Part model, mm, in its own coordinate system. A direction names the side the tool comes from. Coordinates: 2 decimals unless noted, no trailing zeros. Write each loop counter-clockwise with the first axis right and the second up, starting at its lowest first coordinate (ties: lowest second). Pieces come first, ordered by that corner, then holes. Notation, with made-up numbers: (-39.75, 78.25) - (18.25, 78.25) arc R18 cw to (18.25, 84.25) - close; hole circle Ø8 at (54, -38.5). An arc over 180 degrees is marked (long way). Write each question's results on one line, items separated by ' | '.
from build123d import *

# Parameters (mm, degrees)
F0_R     = 5
F1_DEPTH = 50
F3_DEPTH = 10
F4_W     = 15
F4_H     = 15
F4_R     = 5
F5_DEPTH = 10
F6_R     = 5
F7_DEPTH = 2.5
F8_SIZE  = 2.49999


# Not quite as in the source:
# - a fillet or chamfer is up to 0.001 mm smaller than in the source, because OpenCascade refuses the exact size


with BuildPart() as f1:
    # F0 (on Right) → F1 (new body)
    with BuildSketch(Plane.YZ):
        Circle(F0_R)
    extrude(amount=F1_DEPTH)

    # F2 (on face) → F3 (join)
    with BuildSketch(Plane(origin=(0, 0, 0), x_dir=(0, -1, 0), z_dir=(-1, 0, 0))):
        Polygon((11.5200223266, 0.788935313), (5.0767731403, 10.3710996435), (-6.4432491863, 9.5821643305), (-11.5200223266, -0.788935313), (-5.0767731403, -10.3710996435), (6.4432491863, -9.5821643305), align=None)
    extrude(amount=F3_DEPTH)

    # F4 (on face) → F5 (join)
    with BuildSketch(Plane.YZ.offset(50)):
        Rectangle(F4_W, F4_H)
        Circle(F4_R, mode=Mode.SUBTRACT)
    extrude(amount=-F5_DEPTH)

    # F6 (on face) → F7 (join)
    with BuildSketch(Plane.YZ.offset(50)):
        Circle(F6_R)
    extrude(amount=F7_DEPTH)

    # F8 (size 2.5 in the source; OpenCascade refuses exactly that, so slightly less here)
    f8_edges = [f1.edges().sort_by_distance(p)[0] for p in [
        (52.5, -5, 0),
    ]]
    chamfer(f8_edges, length=F8_SIZE)


solid = f1.part
(1) Flat gauge pins, fed straight in: P1, Ø4, axis at y = 1.5, z = -6.5, coming from the +X side; P2, Ø11, axis at x = 43, y = 2, coming from the +Z side; P3, Ø6, axis at y = -2.5, z = -5, coming from the +X side. Where does each tip first touch, or does it go through?
Return value:
P1: stops at x = 50.33 | P2: stops at z = 7.5 | P3: stops at x = 52.41
(2) 3-axis set-ups, long thin cutter, end or side, ignore diameter. For faces 1 (the flat face through (45, -7.5, 0)), 2 (the flat face through (40, -2, 5)), 3 (the flat face through (45, 7.5, 0)): which of +Z, -Z, +X, -X, +Y, -Y reach the whole face in a straight line?
Return value:
face 1: +Z, -Z, +X, -Y | face 2: none | face 3: +Z, -Z, +X, +Y
(3) Wall check: line 1 (X direction, y = 5.5, z = -1.5); line 2 (X direction, y = 9.5, z = -2.75); line 3 (Z direction, x = 46, y = 4.5). Give the ranges that are in metal, low to high. Write a range as from..to.
Return value:
line 1: x = -10..0, 40..50 | line 2: x = -10..0 | line 3: z = -7.5..7.5
(4) Two-plate mould, pull along X, no slides. Class faces 4 (the cylindrical face through (19.72, -1.08, -4.88)), 5 (the conical face through (52, -3, 0)), 6 (the flat face through (-4.93, 0.603, 9.982)), 7 (the flat face through (-10, 0, 0)): released by +X, released by -X, zero draft, split by the parting line, or undercut.
Return value:
face 4: undercut | face 5: released by +X | face 6: zero draft | face 7: released by -X
(5) Saw through at C-C on x = 5. Write the cut outline in (y, z).
Return value:
outline: circle Ø10 at (0, 0)
(6) Saw through at D-D on x = 48. Write the cut outline in (y, z).
Return value:
outline: (-7.5, -7.5) - (7.5, -7.5) - (7.5, 7.5) - (-7.5, 7.5) - close
